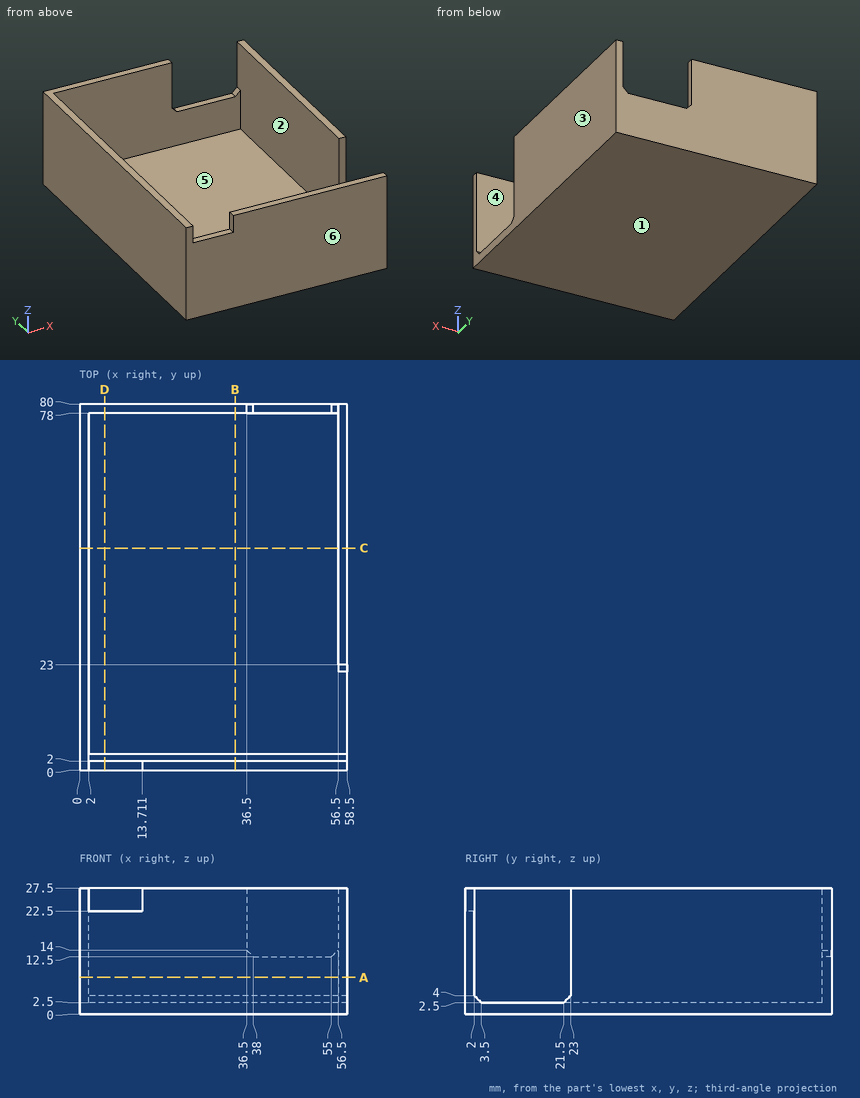
Here's the drawing with two shaded views (mm, measured from the low corner). I have some questions. A direction names the side the tool comes from. Round coordinates to 2 decimals unless told otherwise and drop trailing zeros. Loops run counter-clockwise (first coordinate to the right, second up) from the corner with the lowest first, then second, coordinate; pieces in that order, holes last.
1. Will these pins go through, and if not, where does the flat tip stop? pin 1 (1.6 mm diameter, centred on x = 7.5, y = 1, fed in from +Z); pin 2 (3 mm diameter, centred on x = 33, y = 35.5, fed in from -Z); pin 3 (0.6 mm diameter, centred on x = 45, y = 78.5, fed in from +Z); pin 4 (3 mm diameter, centred on x = 40.5, z = 19.5, fed in from +Y).
Answers:
pin 1: stops at z = 22.5
pin 2: stops at z = 0
pin 3: stops at z = 12.5
pin 4: stops at y = 2
2. For the marked faces 4, 5 and 6, which set-ups out of +Z, -Z, +X, -X, +Y, -Y let a thin tool reach every point of the face, with its end or its side?
Answers:
face 4: +Z, +X
face 5: +Z
face 6: +Z, -Z, +X, -X, -Y
3. Suppose I cut it at B-B, the plane x = 34. Please give me the cut outline in (y, z), and give its area (3 significant figures).
Answers:
outline: (0, 0) - (80, 0) - (80, 27.5) - (78, 27.5) - (78, 2.5) - (3.5, 2.5) - (2, 4) - (2, 27.5) - (0, 27.5) - close
area: 301 mm2
4. If I drill on probe 1 along X at (y, z) = (38, 15.5); probe 2 along Y at (x, z) = (20, 12); probe 3 along Z at (x, y) = (31.5, 45.5), over which ranges is the centre line in solid material (lowest first)?
Answers:
probe 1: x = 0 to 2, 56.5 to 58.5
probe 2: y = 0 to 2, 78 to 80
probe 3: z = 0 to 2.5
5. Suppose I cut it at D-D, the plane x = 5.5. Please give me the cut outline in (y, z), and give its area (3 significant figures).
Answers:
outline: (0, 0) - (80, 0) - (80, 27.5) - (78, 27.5) - (78, 2.5) - (3.5, 2.5) - (2, 4) - (2, 22.5) - (0, 22.5) - close
area: 291 mm2
6. Suppose I cut it at C-C, the plane y = 48.5. Please give me the cut outline in (x, z), and give its area (3 significant figures).
Answers:
outline: (0, 0) - (58.5, 0) - (58.5, 27.5) - (56.5, 27.5) - (56.5, 2.5) - (2, 2.5) - (2, 27.5) - (0, 27.5) - close
area: 246 mm2
7. Thinking about a two-plate mould opening in X: for the marked faces 1, 2 and 3, which applies, released by +X, released by -X, zero draft, split by the parting line, or undercut?
Answers:
face 1: zero draft
face 2: undercut
face 3: released by +X
8. Suppose I cut it at A-A, the plane z = 8. Please give me the cut outline in (x, y), and give its area (3 significant figures).
Answers:
outline: (0, 0) - (58.5, 0) - (58.5, 2) - (2, 2) - (2, 78) - (56.5, 78) - (56.5, 23) - (58.5, 23) - (58.5, 80) - (0, 80) - close
area: 496 mm2
